The listing builds one solid part. Answer for the finished solid, in the listing's coordinates (mm). A direction names the side the tool comes from. Give positions to 0.01 mm unless a question says otherwise; leave off trailing zeros. Write each loop counter-clockwise with the first axis right and the second up, starting at its lowest first coordinate (ties: lowest second). Pieces come first, ordered by that corner, then holes. Notation, with made-up numbers: (-10, 56) - (21, 56) arc R17 ccw to (21, 89) - close; hole circle Ø2 at (-13, 8). An arc over 180 degrees is marked (long way). Return JSON: item names as keys, results as strings.
from build123d import *

# Parameters (mm, degrees)
BOSS_EXTRUDE1_DEPTH     = 25
SKETCH1_3_R             = 30
BOSS_EXTRUDE2_DEPTH     = 40
SKETCH2_W               = 40
SKETCH2_H               = 60
CUT_EXTRUDE1_DEPTH      = 10
CUT_EXTRUDE2_DEPTH      = 108.354552768
CUT_EXTRUDE2_DEPTH_BACK = 108.354552768
SKETCH3_R               = 10
CUT_EXTRUDE3_DEPTH      = 112.803398875
CUT_EXTRUDE3_DEPTH_BACK = 112.803398875


with BuildPart() as part:
    # Sketch1 → Boss-Extrude1 (new body)
    with BuildSketch(Plane(origin=(0, 0, 0), x_dir=(0, 1, 0), z_dir=(0, 0, 1))):
        with BuildLine():
            Line((100, 30), (0, 30))
            ThreePointArc((0, 30), (21.213203436, 21.213203436), (30, 0))
            ThreePointArc((30, 0), (21.213203436, -21.213203436), (0, -30))
            Line((0, -30), (100, -30))
            Line((100, -30), (100, 30))
        make_face()
    extrude(amount=BOSS_EXTRUDE1_DEPTH)

    # Sketch1_3 → Boss-Extrude2 (add)
    with BuildSketch(Plane(origin=(0, 0, 0), x_dir=(0, 1, 0), z_dir=(0, 0, 1))):
        with Locations(Location((0, 0, 0), (0, 0, 270))):
            Circle(SKETCH1_3_R)
    extrude(amount=BOSS_EXTRUDE2_DEPTH)

    # Sketch2 → Cut-Extrude1 (cut)
    with BuildSketch(Plane.XY.offset(25)):
        with Locations((0, 70)):
            Rectangle(SKETCH2_W, SKETCH2_H)
    extrude(amount=-CUT_EXTRUDE1_DEPTH, mode=Mode.SUBTRACT)

    # Sketch3 → Cut-Extrude2 (cut, two sides: drawn at the far end of the back side and taken through both)
    with BuildSketch(Plane.XY.offset(15).offset(-CUT_EXTRUDE2_DEPTH_BACK)):
        with Locations((0, 70)):
            Circle(SKETCH3_R)
    extrude(amount=CUT_EXTRUDE2_DEPTH + CUT_EXTRUDE2_DEPTH_BACK, mode=Mode.SUBTRACT)

    # Sketch4 → Cut-Extrude3 (cut, two sides: drawn at the far end of the back side and taken through both)
    with BuildSketch(Plane.XY.offset(40).offset(-CUT_EXTRUDE3_DEPTH_BACK)):
        with BuildLine():
            Line((-4, 18.456832295), (4, 18.456832295))
            Line((4, 18.456832295), (4, 14.456832295))
            ThreePointArc((4, 14.456832295), (0, -15), (-4, 14.456832295))
            Line((-4, 14.456832295), (-4, 18.456832295))
        make_face()
    extrude(amount=CUT_EXTRUDE3_DEPTH + CUT_EXTRUDE3_DEPTH_BACK, mode=Mode.SUBTRACT)


solid = part.part
Item 1: Flat-ended cylindrical pins translate along their axes: P1, Ø6, axis at x = 23, z = 15.5, coming from the -Y side; P2, Ø5, axis at x = -22, z = 32.5, coming from the +Y side; P3, Ø2.5, axis at x = 0, z = 17.5, coming from the -Y side. Find the tip coordinate at first contact, or state that the pin passes through.
Answer below:
{"P1": "stops at y = -22.36", "P2": "stops at y = 22.8", "P3": "stops at y = -30"}
Item 2: Consider L1, parallel to X at y = 70, z = 6.75; L2, parallel to Y at x = -7, z = 8; L3, parallel to Y at x = -2.5, z = 8. Determine where each line is inside the solid, lowest interval first.
Answer below:
{"L1": "x = -30 to -10, 10 to 30", "L2": "y = -29.17 to -13.27, 13.27 to 62.86, 77.14 to 100", "L3": "y = -29.9 to -14.79, 18.46 to 60.32, 79.68 to 100"}
Item 3: For faces 4 (the face through (0, 36, 0)), 5 (the face through (9, 77, 15)), 6 (the face through (0, 18.457, 20)), 7 (the face through (13.843, -26.615, 24.164)), 8 (the face through (0, 100, 10)), determine the directions among +Z, -Z, +X, -X, +Y, -Y from which every point of the face is accessible in a straight line to the end or side of a thin tool.
Answer below:
{"face 4": "-Z, +X, -X, +Y, -Y", "face 5": "+Z, +Y", "face 6": "+Z, -Z", "face 7": "+Z", "face 8": "+Z, -Z, +X, -X, +Y"}
Item 4: A cutting plane is placed at C-C on z = 36. Determine the outline of the cut face in (x, y), then the cut area to 3 significant figures.
Answer below:
{"outline": "circle Ø60 at (0, 0); hole (-4, 14.46) arc R15 ccw (long way) to (4, 14.46) - (4, 18.46) - (-4, 18.46) - close", "area": "2,090 mm²"}
Item 5: A cutting plane is placed at D-D on y = 34. Determine the outline of the cut face in (x, z), then the cut area to 3 significant figures.
Answer below:
{"outline": "(-30, 0) - (30, 0) - (30, 25) - (-30, 25) - close", "area": "1,500 mm²"}
Item 6: A cutting plane is placed at B-B on x = 0. Determine the outline of the cut face in (y, z), then the cut area to 3 significant figures.
Answer below:
{"outline": "(-30, 0) - (-15, 0) - (-15, 40) - (-30, 40) - close; (18.46, 0) - (60, 0) - (60, 15) - (40, 15) - (40, 25) - (30, 25) - (30, 40) - (18.46, 40) - close; (80, 0) - (100, 0) - (100, 15) - (80, 15) - close", "area": "1,910 mm²"}
Item 7: A cutting plane is placed at A-A on y = 70. Determine the outline of the cut face in (x, z).
Answer below:
{"outline": "(-30, 0) - (-10, 0) - (-10, 15) - (-20, 15) - (-20, 25) - (-30, 25) - close; (10, 0) - (30, 0) - (30, 25) - (20, 25) - (20, 15) - (10, 15) - close"}
Item 8: The mould has two halves that part along Y. Classify faces 1 (the face through (6, 14, 40)), 2 (the face through (-4, 16, 20)), 3 (the face through (0, 40, 20)): +Y half, -Y half, draft (parallel to the pull), parting line (faces both ways), or undercut.
Answer below:
{"face 1": "draft", "face 2": "undercut", "face 3": "+Y half"}
